Geometry check sheet. Reference: the model listing, model coordinates, mm. Face numbers are marked on the shaded views. Round coordinates to 2 decimals unless told otherwise and drop trailing zeros. Order: outer loops, then holes, each group sorted by start corner. A loop starts at its lowest first (then second) coordinate and runs counter-clockwise, first axis right, second up. Notation, with made-up numbers: (28.25, 4.5) - (34.25, 4.5) arc R19 cw to (34.25, 32.5) - close; hole circle Ø7 at (67, 28). An arc over 180 degrees is marked (long way). Answer as CSV lines item,"result". Start each with the question number.
```python
from build123d import *

# Parameters (mm, degrees)
BOSS_EXTRUDE1_START = -304.8
SKETCH2_R           = 76.2
SKETCH2_R_2         = 73.2
BOSS_EXTRUDE1_DEPTH = 304.8
SKETCH3_R           = 126.460441223
CUT_EXTRUDE1_DEPTH  = 30


with BuildPart() as part:
    # Sketch1 → Revolve3 (revolve)
    with BuildSketch(Plane.XY, mode=Mode.PRIVATE) as revolve3_sk:
        with BuildLine():
            Line((78.16, 0.555796301), (78.16, 150.555796301))
            add(Edge.make_bspline(
                [(0, 400), (0.211335822, 399.688125951), (0.635814895, 399.059576984), (1.538100901, 397.718447682), (2.522216135, 396.240558988), (3.505644669, 394.750882712), (4.501021999, 393.230772914), (5.482794304, 391.717940875), (6.460002487, 390.1990457), (7.436503499, 388.667903295), (8.412102246, 387.124567018), (16.491350088, 374.228806244), (28.348045348, 353.344444451), (42.541088503, 323.752786496), (57.529234868, 282.998416237), (68.449765851, 242.872883661), (74.109605793, 210.076821303), (76.655852831, 184.808563), (77.518465345, 170.067485067), (77.680444963, 166.851372886), (77.80019329, 164.105278722), (77.872037245, 162.29067577), (77.936311693, 160.485721023), (77.993377873, 158.683168323), (78.043426294, 156.866740105), (78.085914262, 155.082628956), (78.121127528, 153.306463123), (78.145475643, 151.691137071), (78.155577952, 150.932503957), (78.16, 150.555796301)],
                knots=[0.082616428, 0.082616428, 0.082616428, 0.082616428, 0.082616428, 0.088299706, 0.093982984, 0.099666263, 0.105349541, 0.111032819, 0.116716097, 0.122399375, 0.128082653, 0.133891142, 0.139699631, 0.313954311, 0.430124092, 0.546293874, 0.685697612, 0.836718331, 0.848335309, 0.865760775, 0.871569264, 0.877252541, 0.882935819, 0.888619096, 0.894302373, 0.899985651, 0.905668928, 0.911352205, 0.917035483, 0.917035483, 0.917035483, 0.917035483, 0.917035483], degree=4))
            Line((0, 400), (0, 396.489212171))
            add(Edge.make_bspline(
                [(0, 396.489212171), (0.033950421, 396.438447854), (0.270297298, 396.084910627), (0.687269239, 395.458986868), (1.248256795, 394.612262217), (1.999478916, 393.472916562), (3.322990367, 391.451301251), (5.182734219, 388.567106013), (9.592096746, 381.590651127), (18.79448878, 366.267083026), (36.794305295, 332.203153979), (57.076508975, 280.924103704), (69.684732597, 227.240425292), (74.343019544, 188.995844434), (75.530951553, 171.160960641), (75.891349594, 162.915707977), (76.010098219, 159.486050775), (76.07694035, 157.070550778), (76.110246707, 155.706228582), (76.132780312, 154.690650434), (76.153251031, 153.650034533), (76.172421756, 152.520648044), (76.189027326, 151.409738144), (76.196427769, 150.847643517), (76.2, 150.54427492)],
                knots=[0.091851146, 0.091851146, 0.091851146, 0.091851146, 0.092394266, 0.095653545, 0.098912824, 0.102172103, 0.108690662, 0.121727778, 0.134764895, 0.186913362, 0.291210296, 0.499804164, 0.708398032, 0.812694966, 0.864843432, 0.877880549, 0.890917666, 0.897436224, 0.900695504, 0.903954783, 0.907214062, 0.910473341, 0.91373262, 0.916991899, 0.916991899, 0.916991899, 0.916991899], degree=3))
            Line((76.2, 150.54427492), (76.2, 0.555796301))
            Line((76.2, 0.555796301), (78.16, 0.555796301))
        make_face()
    revolve(revolve3_sk.sketch.rotate(Axis((0, -198.817850362, 0), (0, -1, 0)), 90), axis=Axis((0, -198.817850362, 0), (0, -1, 0)))

    # Sketch2 → Boss-Extrude1 (add)
    with BuildSketch(Plane(origin=(0, 150.555796301, 0), x_dir=(1, 0, 0), z_dir=(0, 1, 0)).offset(BOSS_EXTRUDE1_START)):
        with Locations(Location((0, 0, 0), (0, 0, 270))):
            Circle(SKETCH2_R)
        with Locations(Location((0, 0, 0), (0, 0, 270))):
            Circle(SKETCH2_R_2, mode=Mode.SUBTRACT)
    extrude(amount=BOSS_EXTRUDE1_DEPTH)

    # Sketch3 → Cut-Extrude1 (cut)
    with BuildSketch(Plane(origin=(0, 400, 0), x_dir=(-1, 0, 0), z_dir=(0, -1, 0))):
        Circle(SKETCH3_R)
    extrude(amount=CUT_EXTRUDE1_DEPTH, mode=Mode.SUBTRACT)


solid = part.part
```
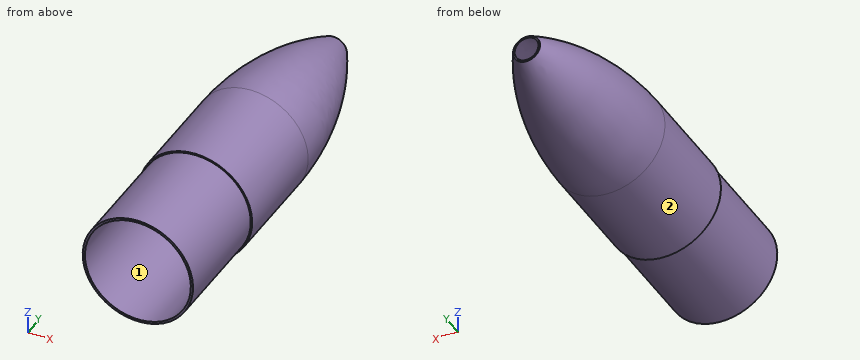
1. Draft check along X on the marked faces 1 and 2. Enter one of: released by +X, released by -X, zero draft, split by the parting line, or undercut.
2. Section check A-A on y = 127. Record the boundary of the cut face in (x, z), plus the area to 3 significant figures.
3. Thickness scan on probe 1 along X at (y, z) = (3, 0); probe 2 along X at (y, z) = (-1, 0); probe 3 along Z at (x, y) = (59, 70). Record the ranges inside material, lowest first.
4. Section check B-B on y = -40.5. Record the boundary of the cut face in (x, z).
5. Go/stop test with flat-tipped pins: pin 1 Ø1 at (x, y) = (52, 198) entering from +Z; pin 2 Ø6 at (x, z) = (-36, -19.5) entering from +Y; pin 3 Ø4 at (y, z) = (203.5, 47.5) entering from +X. Record where each tip stops, or that it passes through.
Numbers:
1,face 1,"undercut"
1,face 2,"split by the parting line"
2,outline,"circle Ø156.32 at (0, 0); hole circle Ø146.4 at (0, 0)"
2,area,"2,360 mm2"
3,probe 1,"x = -78.16 to -73.2, 73.2 to 78.16"
3,probe 2,"x = -76.2 to -73.2, 73.2 to 76.2"
3,probe 3,"z = -51.26 to -43.33, 43.33 to 51.26"
4,outline,"circle Ø152.4 at (0, 0); hole circle Ø146.4 at (0, 0)"
5,pin 1,"stops at z = 54.69"
5,pin 2,"stops at y = 332.15"
5,pin 3,"stops at x = 58.95"
